CAD build for the part. Positions are in the model's coordinates, mm. A direction names the side the tool comes from. Give positions to 0.01 mm unless a question says otherwise; leave off trailing zeros. Write each loop counter-clockwise with the first axis right and the second up, starting at its lowest first coordinate (ties: lowest second). Pieces come first, ordered by that corner, then holes. Notation, with made-up numbers: M 12,-36 L 20,-36 A13 cw 20,-31 Z; hole C -35.5,62.25 d4. An arc over 180 degrees is marked long. One line per question, with ' | ' between items. Start each with the question number.
1. Which spindle directions (+Z, -Z, +X, -X, +Y, -Y) get a long thin tool onto all of the face, cutting with end or side? Do faces 1 (the face through (-0.1, -8, 2.2)), 2 (the face through (2, -2, 5)), 3 (the face through (-1, -4, -3)), 4 (the face through (2, 0, 5)). Say none if no direction does.
2. Pull direction Z, two halves, no side cores. Call faces 5 (the face through (-4.88, 1.97, -1.08)), 6 (the face through (-2.3, 6, -0.2)), 7 (the face through (0, -1, 2)): released by +Z, released by -Z, zero draft, split by the parting line, or undercut.
3. Wall check: L1, parallel to X at y = -2.75, z = 0; L2, parallel to Y at x = 7.75, z = -2.25; L3, parallel to Y at x = 0, z = -2.95. Give the ranges that are in metal, low to high.
4. Cut at B-B, the plane x = 0. Count the separate pieces of the cut face and the enclosed holes in it, then the cut area to 3 significant figures.
5. Flat gauge pins, fed straight in: pin 1 (1 mm diameter, centred on x = 5, y = 1.5, fed in from +Z); pin 2 (2 mm diameter, centred on x = -9.5, z = -2.5, fed in from -Y); pin 3 (4 mm diameter, centred on y = -4.5, z = -2.5, fed in from +X). Where does each tip first touch, or does it go through?
6. Cut at D-D, the plane y = -4. Write the cut outline in (x, z).
7. Cut at C-C, the plane y = 2. Write the cut outline in (x, z), then the cut area to 3 significant figures.
```python
from build123d import *

# Parameters (mm, degrees)
SKETCH_1_R          = 5
EXTRUDE_1_DEPTH     = 4
SKETCH_2_R          = 12
EXTRUDE_2_DEPTH     = 2
EXTRUDE_START       = 2
SKETCH_3_R          = 12
EXTRUDE_3_DEPTH     = 2
EXTRUDE_START_2     = 6
SKETCH_4_R          = 5
EXTRUDE_4_DEPTH     = 6
SKETCH_5_R          = 2
CUT_EXTRUDE_1_DEPTH = 23
FILLET_2_R          = 1
SKETCH_6_R          = 1
CUT_EXTRUDE_2_DEPTH = 19.761663039


with BuildPart() as part:
    # 草图1 → 凸台-拉伸1 (new body)
    with BuildSketch(Plane(origin=(0, 0, 0), x_dir=(1, 0, 0), z_dir=(0, 1, 0))):
        with Locations(Location((0, 0, 0), (0, 0, 270))):
            Circle(SKETCH_1_R)
    extrude(amount=EXTRUDE_1_DEPTH)

    # 草图2 → 凸台-拉伸2 (add)
    with BuildSketch(Plane(origin=(0, 4, 0), x_dir=(1, 0, 0), z_dir=(0, 1, 0))):
        with Locations(Location((0, 0, 0), (0, 0, 270))):
            Circle(SKETCH_2_R)
    extrude(amount=EXTRUDE_2_DEPTH)

    # 草图3 → 凸台-拉伸3 (add)
    with BuildSketch(Plane.XZ.offset(EXTRUDE_START)):
        with Locations(Location((0, 0, 0), (0, 0, 90))):
            Circle(SKETCH_3_R)
    extrude(amount=-EXTRUDE_3_DEPTH)

    # 草图4 → 凸台-拉伸4 (add)
    with BuildSketch(Plane(origin=(0, -2, 0), x_dir=(-1, 0, 0), z_dir=(0, -1, 0)).offset(EXTRUDE_START_2)):
        with Locations(Location((0, 0, 0), (0, 0, 270))):
            Circle(SKETCH_4_R)
    extrude(amount=-EXTRUDE_4_DEPTH)

    # 草图5 → 切除-拉伸1 (cut, through all)
    with BuildSketch(Plane.XZ.offset(8)):
        with Locations(Location((0, 0, 0), (0, 0, 270))):
            Circle(SKETCH_5_R)
    extrude(amount=-CUT_EXTRUDE_1_DEPTH, mode=Mode.SUBTRACT)

    # 圆角2
    fillet_2_edges = [part.edges().sort_by_distance(p)[0] for p in [
        (0, -2, -12),
        (0, 4, -12),
        (0, 6, -12),
        (0, 0, -12),
    ]]
    fillet(fillet_2_edges, radius=FILLET_2_R - 0.0001)  # a hair under: the kernel refuses the full size

    # 草图6 → 切除-拉伸2 (cut, through all)
    with BuildSketch(Plane.XY):
        with Locations(Location((0, -4, 0), (0, 0, 90))):
            Circle(SKETCH_6_R)
    extrude(amount=-CUT_EXTRUDE_2_DEPTH, mode=Mode.SUBTRACT)


solid = part.part
```
Here are the results:
1) face 1: +Z, -Z, +X, -X, -Y | face 2: -Y | face 3: -Z | face 4: none
2) face 5: split by the parting line | face 6: zero draft | face 7: undercut
3) L1: -5 to -2, 2 to 5 | L2: -2 to 0, 4 to 6 | L3: -8 to -5, -3 to 6
4) separate pieces: 3 | enclosed holes: 0 | area: 132 mm^2
5) pin 1: z = 2.18 | pin 2: y = -2 | pin 3: x = 4.97
6) outline: M -1,-4.9 L -1,-1.73 A2 cw long 1,-1.73 L 1,-4.9 A5 ccw long Z
7) outline: C 0,0 d10; hole C 0,0 d4 | area: 66.0 mm^2
